```python
from build123d import *

# Parameters (mm, degrees)
SKETCH1_W           = 103.11
SKETCH1_H           = 90.78
BOSS_EXTRUDE1_DEPTH = 6.65
SKETCH2_W           = 9.01
SKETCH2_H           = 3.54
BOSS_EXTRUDE2_DEPTH = 10.65
BOSS_EXTRUDE3_DEPTH = 10.18
SKETCH4_R           = 3.26
CUT_EXTRUDE1_DEPTH  = 10.18
SKETCH6_R           = 1.25
BOSS_EXTRUDE4_DEPTH = 9.18
SKETCH7_W           = 18
SKETCH7_H           = 14.17
BOSS_EXTRUDE5_DEPTH = 6
SKETCH8_W           = 16.5
SKETCH8_H           = 4.82
CUT_EXTRUDE2_DEPTH  = 9
SKETCH9_W           = 15.72
SKETCH9_H           = 14
BOSS_EXTRUDE6_DEPTH = 15
SKETCH10_W          = 12.25
SKETCH10_H          = 5.08
CUT_EXTRUDE3_DEPTH  = 7.5
SKETCH12_W          = 15.72
SKETCH12_H          = 13.964065117
BOSS_EXTRUDE7_DEPTH = 15
SKETCH13_W          = 12.25
SKETCH13_H          = 5.08
CUT_EXTRUDE4_DEPTH  = 7.5


with BuildPart() as part:
    # Sketch1 → Boss-Extrude1 (new body)
    with BuildSketch(Plane(origin=(0, 0, 0), x_dir=(1, 0, 0), z_dir=(0, 1, 0))):
        Rectangle(SKETCH1_W, SKETCH1_H)
    extrude(amount=BOSS_EXTRUDE1_DEPTH)

    # Sketch2 → Boss-Extrude2 (add)
    with BuildSketch(Plane(origin=(0, 6.65, 0), x_dir=(1, 0, 0), z_dir=(0, 1, 0))):
        with Locations((-43.92, -43.350225169)):
            Rectangle(SKETCH2_W, SKETCH2_H)
    extrude(amount=BOSS_EXTRUDE2_DEPTH)

    # Sketch3 → Boss-Extrude3 (add)
    with BuildSketch(Plane(origin=(0, 0, 41.580225169), x_dir=(-1, 0, 0), z_dir=(0, 0, -1))):
        with BuildLine():
            Line((39.415, 6.65), (39.415, 11.078180036))
            ThreePointArc((39.415, 11.078180036), (43.92, 15.856037514), (48.425, 11.078180036))
            Line((48.425, 11.078180036), (48.425, 6.65))
            Line((48.425, 6.65), (39.415, 6.65))
        make_face()
    extrude(amount=BOSS_EXTRUDE3_DEPTH)

    # Sketch4 → Cut-Extrude1 (cut)
    with BuildSketch(Plane.XY.offset(45.120225169)):
        with Locations((-43.925, 12.286078197)):
            Circle(SKETCH4_R)
    extrude(amount=-CUT_EXTRUDE1_DEPTH, mode=Mode.SUBTRACT)

    # Sketch6 → Boss-Extrude4 (add)
    with BuildSketch(Plane.XY.offset(34.940225169)):
        with Locations((-43.925906585, 12.376780876)):
            Circle(SKETCH6_R)
    extrude(amount=BOSS_EXTRUDE4_DEPTH)

    # Sketch7 → Boss-Extrude5 (add)
    with BuildSketch(Plane(origin=(0, 6.65, 0), x_dir=(1, 0, 0), z_dir=(0, 1, 0))):
        with Locations((-27.007208725, -38.305)):
            Rectangle(SKETCH7_W, SKETCH7_H)
    extrude(amount=BOSS_EXTRUDE5_DEPTH)

    # Sketch8 → Cut-Extrude2 (cut)
    with BuildSketch(Plane.XY.offset(45.39)):
        with Locations((-26.982569048, 9.597847623)):
            Rectangle(SKETCH8_W, SKETCH8_H)
    extrude(amount=-CUT_EXTRUDE2_DEPTH, mode=Mode.SUBTRACT)

    # Sketch9 → Boss-Extrude6 (add)
    with BuildSketch(Plane(origin=(0, 6.65, 0), x_dir=(1, 0, 0), z_dir=(0, 1, 0))):
        with Locations((-5.847208725, -38.39)):
            Rectangle(SKETCH9_W, SKETCH9_H)
    extrude(amount=BOSS_EXTRUDE6_DEPTH)

    # Sketch10 → Cut-Extrude3 (cut)
    with BuildSketch(Plane.XY.offset(45.39)):
        with Locations((-5.831324622, 18.0957287)):
            Rectangle(SKETCH10_W, SKETCH10_H)
        with Locations((-5.831324622, 9.615530297)):
            Rectangle(SKETCH10_W, SKETCH10_H)
    extrude(amount=-CUT_EXTRUDE3_DEPTH, mode=Mode.SUBTRACT)

    # Sketch12 → Boss-Extrude7 (add)
    with BuildSketch(Plane(origin=(0, 6.65, 0), x_dir=(1, 0, 0), z_dir=(0, 1, 0))):
        with Locations((12.572791275, -38.407967442)):
            Rectangle(SKETCH12_W, SKETCH12_H)
    extrude(amount=BOSS_EXTRUDE7_DEPTH)

    # Sketch13 → Cut-Extrude4 (cut)
    with BuildSketch(Plane.XY.offset(45.39)):
        with Locations((12.656700486, 17.962850519)):
            Rectangle(SKETCH13_W, SKETCH13_H)
        with Locations((12.656700486, 9.482652117)):
            Rectangle(SKETCH13_W, SKETCH13_H)
    extrude(amount=-CUT_EXTRUDE4_DEPTH, mode=Mode.SUBTRACT)


solid = part.part
```
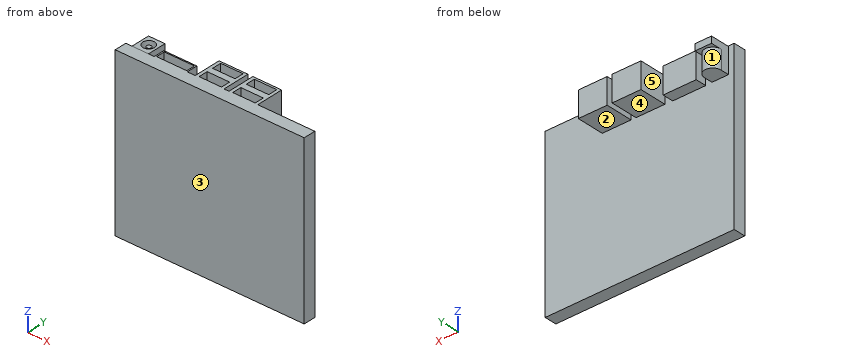
Design review of the part built by this model. Coordinates are the model's own, in mm. Face numbers are marked on the shaded views. A direction names the side the tool comes from. Give positions to 0.01 mm unless a question says otherwise; leave off trailing zeros. Write each loop counter-clockwise with the first axis right and the second up, starting at its lowest first coordinate (ties: lowest second). Pieces come first, ordered by that corner, then holes. Notation, with made-up numbers: (-26, -16) -> (-10, -16) arc R24 ccw to (-10, 5) -> close; hole circle Ø4 at (45, 17.5). An arc over 180 degrees is marked (long way). Answer in a Markdown table with one row per item.
(1) Consider section D-D (x = -43.92). State the section outline as (y, z) points.
Results:
| item | result |
|---|---|
| outline | (0, -45.39) -> (6.65, -45.39) -> (6.65, 31.4) -> (15.86, 31.4) -> (15.86, 41.58) -> (17.3, 41.58) -> (17.3, 45.12) -> (15.55, 45.12) -> (15.55, 34.94) -> (13.63, 34.94) -> (13.63, 44.12) -> (11.13, 44.12) -> (11.13, 34.94) -> (9.03, 34.94) -> (9.03, 45.12) -> (6.65, 45.12) -> (6.65, 45.39) -> (0, 45.39) -> close |
(2) Consider section B-B (z = -4.5). State the section outline as (x, y) points (3 decimals), then the cut area to 3 significant figures.
Results:
| item | result |
|---|---|
| outline | (-51.555, 0) -> (51.555, 0) -> (51.555, 6.65) -> (-51.555, 6.65) -> close |
| area | 686 mm2 |
(3) Consider section C-C (x = -24.5). State the section outline as (y, z) points.
Results:
| item | result |
|---|---|
| outline | (0, -45.39) -> (6.65, -45.39) -> (6.65, 31.22) -> (12.65, 31.22) -> (12.65, 45.39) -> (12.01, 45.39) -> (12.01, 36.39) -> (7.19, 36.39) -> (7.19, 45.39) -> (0, 45.39) -> close |
(4) Clearance check with flat-ended pins moving along their axes: pin 1 (1.5 mm diameter, centred on x = 14.5, y = 9.5, fed in from +Z); pin 2 (7 mm diameter, centred on y = 15, z = 37.5, fed in from -X); pin 3 (2.5 mm diameter, centred on x = -45.5, y = 13, fed in from -Z); pin 4 (2 mm diameter, centred on y = 8.5, z = -0.5, fed in from -X). State where each tip first meets the part, or that it passes through.
Results:
| item | result |
|---|---|
| pin 1 | z = 37.89 |
| pin 2 | x = -48.43 |
| pin 3 | z = 31.4 |
| pin 4 | through |
(5) Consider section A-A (x = -3). State the section outline as (y, z) points.
Results:
| item | result |
|---|---|
| outline | (0, -45.39) -> (6.65, -45.39) -> (6.65, 31.39) -> (21.65, 31.39) -> (21.65, 45.39) -> (20.64, 45.39) -> (20.64, 37.89) -> (15.56, 37.89) -> (15.56, 45.39) -> (12.16, 45.39) -> (12.16, 37.89) -> (7.08, 37.89) -> (7.08, 45.39) -> (0, 45.39) -> close |
(6) Mouldability with a two-part tool opening along X and no side actions: class the marked faces 1 and 2 as +X half, -X half, draft (parallel to the pull), parting line (faces both ways), or undercut.
Results:
| item | result |
|---|---|
| face 1 | undercut |
| face 2 | draft |
(7) For the marked faces 3, 4 and 5, list the 3-axis set-ups (+Z, -Z, +X, -X, +Y, -Y) from which the entire face can be reached by the end or side of a thin tool; tool diameter is ignored.
Results:
| item | result |
|---|---|
| face 3 | +Z, -Z, +X, -X, -Y |
| face 4 | -Z, +X, +Y |
| face 5 | +Z, -Z, +Y |
(8) To check wall thickness, follow probe 1 along Y at (x, z) = (-46.5, -24); probe 2 along X at (y, z) = (17.5, 34); probe 3 along Z at (x, y) = (5, 15.75). State the ranges of each line that lie inside material, in increasing order.
Results:
| item | result |
|---|---|
| probe 1 | 0 to 6.65 |
| probe 2 | -13.71 to 2.01, 4.71 to 20.43 |
| probe 3 | 31.43 to 45.39 |
